Autodesk Inventor part; units mm, degrees
ref_plane "YZ Plane" through (0, 0, 0) normal (1, 0, 0) x (0, 1, 0)
ref_plane "XZ Plane" through (0, 0, 0) normal (0, 1, 0) x (-1, 0, 0)
ref_plane "XY Plane" through (0, 0, 0) normal (0, 0, 1) x (1, 0, 0)
sketch "Sketch1" plane through (0, 0, 0) normal (0, 1, 0) x (-1, 0, 0)
  circle A0 centre (0, 0) radius 190.5
  circle A1 centre (0, 0) radius 60.325
  dimension "d0" = 381
  dimension "d1" = 120.65
extrude "Extrusion1" add sketch "Sketch1" along normal blind 12.7
sketch "Sketch2" plane through (0, 12.7, 0) normal (0, 1, 0) x (1, 0, 0)
  line L0 (-142.875, 63.5) -> (-136.525, 63.5)
  line L1 (-136.525, 63.5) -> (-136.525, 50.8)
  line L2 (-136.525, 50.8) -> (-142.875, 50.8)
  line L3 (-142.875, 50.8) -> (-142.875, 63.5)
  line L4 (-136.525, 50.8) -> (-136.525, -50.8) construction
  line L5 (-111.125, 50.8) -> (-212.725, 50.8) construction
  line L6 (-136.525, -50.8) -> (-142.875, -50.8)
  line L7 (-142.875, -50.8) -> (-142.875, -38.1)
  line L8 (-142.875, -38.1) -> (-136.525, -38.1)
  line L9 (-136.525, -38.1) -> (-136.525, -50.8)
  line L10 (-136.525, 0) -> (-60.325, 0) construction
  line L11 (-136.525, 0) -> (-60.325, 0) construction
  circle A0 centre (0, 0) radius 85.725 construction
  line L12 (0, 0) -> (-85.725, 0) construction
  dimension "d4" = 6.35
  dimension "d5" = 12.7
  dimension "d6" = 101.6
  dimension "d7" = 90
  dimension "d8" = 6.35
  dimension "d9" = 12.7
  dimension "d10" = 76.2
  dimension "d11" = 0
extrude "Extrusion2" cut sketch "Sketch2" against normal through all
sketch "Sketch3" plane through (0, 12.7, 0) normal (0, 1, 0) x (1, 0, 0)
  circle A0 centre (0, 0) radius 157.48 construction
  circle A1 centre (-157.48, 0) radius 3.9687
  circle A2 centre (-78.74, -136.3817) radius 3.9687
  circle A3 centre (78.74, -136.3817) radius 3.9687
  circle A4 centre (157.48, 0) radius 3.9687
  circle A5 centre (78.74, 136.3817) radius 3.9687
  circle A6 centre (-78.74, 136.3817) radius 3.9687
  dimension "d16" = 314.96
  dimension "d17" = 7.9375
  dimension "d18" = 360
extrude "Extrusion3" cut sketch "Sketch3" against normal through all
sketch "Sketch4" plane through (0, 12.7, 0) normal (0, 1, 0) x (1, 0, 0)
  line L0 (0, 0) -> (0, -177.8) construction
  line L1 (0, 0) -> (177.8, 0) construction
  circle A0 centre (0, -177.8) radius 3.81
  circle A1 centre (153.9793, -88.9) radius 3.81
  circle A2 centre (153.9793, 88.9) radius 3.81
  circle A3 centre (0, 177.8) radius 3.81
  circle A4 centre (-153.9793, 88.9) radius 3.81
  circle A5 centre (-153.9793, -88.9) radius 3.81
  dimension "d21" = 177.8
  dimension "d22" = 90
  dimension "d23" = 7.62
  dimension "d26" = 360
extrude "Extrusion4" cut sketch "Sketch4" against normal through all
sketch "Sketch5" plane through (0, 12.7, 0) normal (0, 1, 0) x (1, 0, 0)
  circle A0 centre (-157.48, 0) radius 3.9687
  circle A1 centre (-157.48, 0) radius 12.7
  point P0 (0, 0)
  dimension "d30" = 25.4
extrude "Extrusion5" cut sketch "Sketch5" against normal through all
sketch "Sketch6" plane through (0, 12.7, 0) normal (0, 1, 0) x (1, 0, 0)
  circle A0 centre (-157.48, 0) radius 12.7
  line L0 (-157.48, 12.7) -> (-93.98, 12.7)
  line L1 (-93.98, 12.7) -> (-93.98, -12.7)
  line L2 (-93.98, -12.7) -> (-157.48, -12.7)
  line L3 (-157.48, -12.7) -> (-157.48, 12.7)
  point P0 (0, 0)
  dimension "d33" = 63.5
extrude "Extrusion6" cut sketch "Sketch6" against normal through all contours A0 L3 | A0 L0 L1 L2 picked at (-153.2467, 0)
equation "\"d4\" = d8"
properties part number "Turntable Mid" material "PVC-Piping"
Read the model definition and answer for the solid it produces. Units are mm, in the model's axes. A direction names the side the tool comes from. Give positions to 0.01 mm unless a question says otherwise; leave off trailing zeros. Loops run counter-clockwise (first coordinate to the right, second up) from the corner with the lowest first, then second, coordinate; pieces in that order, holes last. Notation, with made-up numbers: M 25,79 L 58,79 A26 cw 58,111 Z; hole C 16.5,75 d5. An arc over 180 degrees is marked long. Write each question's results on one line, items separated by ' | '.
1. Section B-B on y = 10.25 is taken. State how many separate pieces and enclosed holes the cut face has, plus the area to 3 significant figures.
Values:
separate pieces: 1 | enclosed holes: 15 | area: 100,000 mm^2
2. Section D-D on x = 137 is taken. Give the vertices of the cut face in (y, z), plus the area to 3 significant figures.
Values:
outline: M 0,-132.37 L 12.7,-132.37 L 12.7,132.37 L 0,132.37 Z | area: 3,360 mm^2
3. The mould has two halves that part along X. Classify faces 1 (the face through (45, 12.7, 45)), 2 (the face through (151.17, 6.26, 115.92)), 3 (the face through (-93.98, 6, 0)): pulls with the +X half, pulls with the -X half, needs draft (parallel to the pull), parting line crosses it, or undercut.
Values:
face 1: needs draft | face 2: parting line crosses it | face 3: undercut
4. Section C-C on z = -33 is taken. Give the vertices of the cut face in (x, y).
Values:
outline: M -187.62,0 L -50.5,0 L -50.5,12.7 L -187.62,12.7 Z; M 50.5,0 L 187.62,0 L 187.62,12.7 L 50.5,12.7 Z
5. Given pin 1 (6 mm diameter, centred on x = 153.98, z = 88.9, fed in from +Y); pin 2 (6.5 mm diameter, centred on y = 6, z = 46.5, fed in from -X); pin 3 (5 mm diameter, centred on x = -140, y = 6.5, fed in from -Z); pin 4 (1.5 mm diameter, centred on y = 5, z = -12, fed in from -X), each flat-ended and moving along its own axis, determine where each tip first touches the part or whether it passes through.
Values:
pin 1: passes through | pin 2: stops at x = -185.53 | pin 3: stops at z = -131.85 | pin 4: stops at x = -190.17
6. Section A-A on x = -33 is taken. Give the vertices of the cut face in (y, z), plus the area to 3 significant figures.
Values:
outline: M 0,-187.62 L 12.7,-187.62 L 12.7,-50.5 L 0,-50.5 Z; M 0,50.5 L 12.7,50.5 L 12.7,187.62 L 0,187.62 Z | area: 3,480 mm^2
7. Straight lines are drawn through the part: line 1 (Z direction, x = 0, y = 5) (3 decimals); line 2 (Z direction, x = 157.48, y = 7.75); line 3 (X direction, y = 11.5, z = -91). For each, find the intervals that lie inside material, in ascending order. Write a range as [from, to].
Values:
line 1: z = [-190.5, -181.61], [-173.99, -60.325], [60.325, 173.99], [181.61, 190.5] | line 2: z = [-107.19, -90.4], [-87.4, -3.97], [3.97, 87.4], [90.4, 107.19] | line 3: x = [-167.36, -157.16], [-150.8, 150.8], [157.16, 167.36]
8. A tool of negligible diameter and unlimited length cuts with its end or side. For faces 4 (the face through (45, 0, 45)), 5 (the face through (-126, 6, -12.7)), from which of +Z, -Z, +X, -X, +Y, -Y can it reach the whole face along a straight path? Write none if from no direction.
Values:
face 4: +Z, -Z, +X, -X, -Y | face 5: +Y, -Y
